The drawing under review shows one solid part. Ordinate dimensions are in mm from its lowest x, y, z. A direction names the side the tool comes from. Coordinates: 2 decimals unless noted, no trailing zeros. Write each loop counter-clockwise with the first axis right and the second up, starting at its lowest first coordinate (ties: lowest second). Pieces come first, ordered by that corner, then holes.
Q1. To check wall thickness, follow probe 1 along X at (y, z) = (8.5, 35); probe 2 along Y at (x, z) = (6, 24). State the ranges of each line that lie inside material, in increasing order.
Q2. Add section A-A, the plane y = 5.5. Give the boundary of the cut face in (x, z).
Q3. Machinability: for the marked faces 1, 2 and 3, which of the approach directions +Z, -Z, +X, -X, +Y, -Y give a long, thin tool a straight path to every point of the face, cutting with its end or side? Answer none if there is none.
Q4. Add section C-C, the plane x = 22. Give the boundary of the cut face in (y, z), plus the area to 3 significant figures.
Q5. Add section D-D, the plane y = 33.5. Give the boundary of the cut face in (x, z), plus the area to 3 significant figures.
Q6. Add section B-B, the plane z = 22.5. Give the boundary of the cut face in (x, y), plus the area to 3 significant figures.
Q7. Clearance check with flat-ended pins moving along their axes: pin 1 Ø22 at (x, z) = (9, 26) entering from +Y; pin 2 Ø4.5 at (x, z) = (20.5, 28.5) entering from -Y; pin 3 Ø6 at (y, z) = (35, 28) entering from -X. State where each tip first meets the part, or that it passes through.
Q8. The part is to be moulded in two halves that separate along X. For the marked faces 4, 5 and 6, say which applies: +X half, -X half, draft (parallel to the pull), parting line (faces both ways), or undercut.
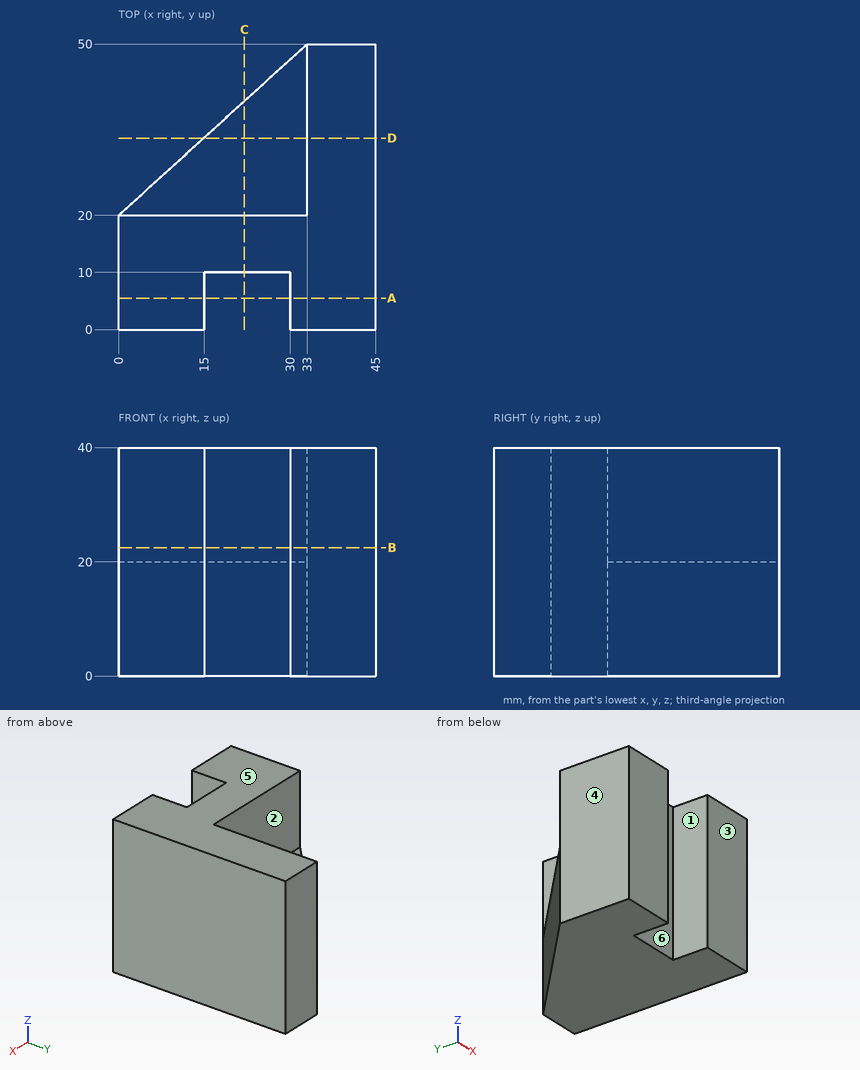
Here are the results:
1. probe 1: x = 0 to 15, 30 to 45
1. probe 2: y = 0 to 20
2. outline: (0, 0) - (15, 0) - (15, 40) - (0, 40) - close; (30, 0) - (45, 0) - (45, 40) - (30, 40) - close
3. face 1: +Z, -Z, -Y
3. face 2: +Z, -X, +Y
3. face 3: +Z, -Z, +X, -X, -Y
4. outline: (10, 0) - (40, 0) - (40, 20) - (20, 20) - (20, 40) - (10, 40) - close
4. area: 800 mm2
5. outline: (14.85, 0) - (45, 0) - (45, 40) - (33, 40) - (33, 20) - (14.85, 20) - close
5. area: 843 mm2
6. outline: (0, 0) - (15, 0) - (15, 10) - (30, 10) - (30, 0) - (45, 0) - (45, 50) - (33, 50) - (33, 20) - (0, 20) - close
6. area: 1,110 mm2
7. pin 1: stops at y = 36.56
7. pin 2: stops at y = 10
7. pin 3: stops at x = 33
8. face 4: -X half
8. face 5: draft
8. face 6: undercut
